The figure shows three views and two pictorial views of one solid part (mm, origin at its lowest corner). Answer the questions. A direction names the side the tool comes from. Round coordinates to 2 decimals unless told otherwise and drop trailing zeros. Order: outer loops, then holes, each group sorted by start corner. A loop starts at its lowest first (then second) coordinate and runs counter-clockwise, first axis right, second up. Notation, with made-up numbers: (28, 11) - (80, 11) arc R15 cw to (80, 39) - close; hole circle Ø6 at (-12, -26.75). An arc over 180 degrees is marked (long way). Answer in a Markdown table with one row per item.
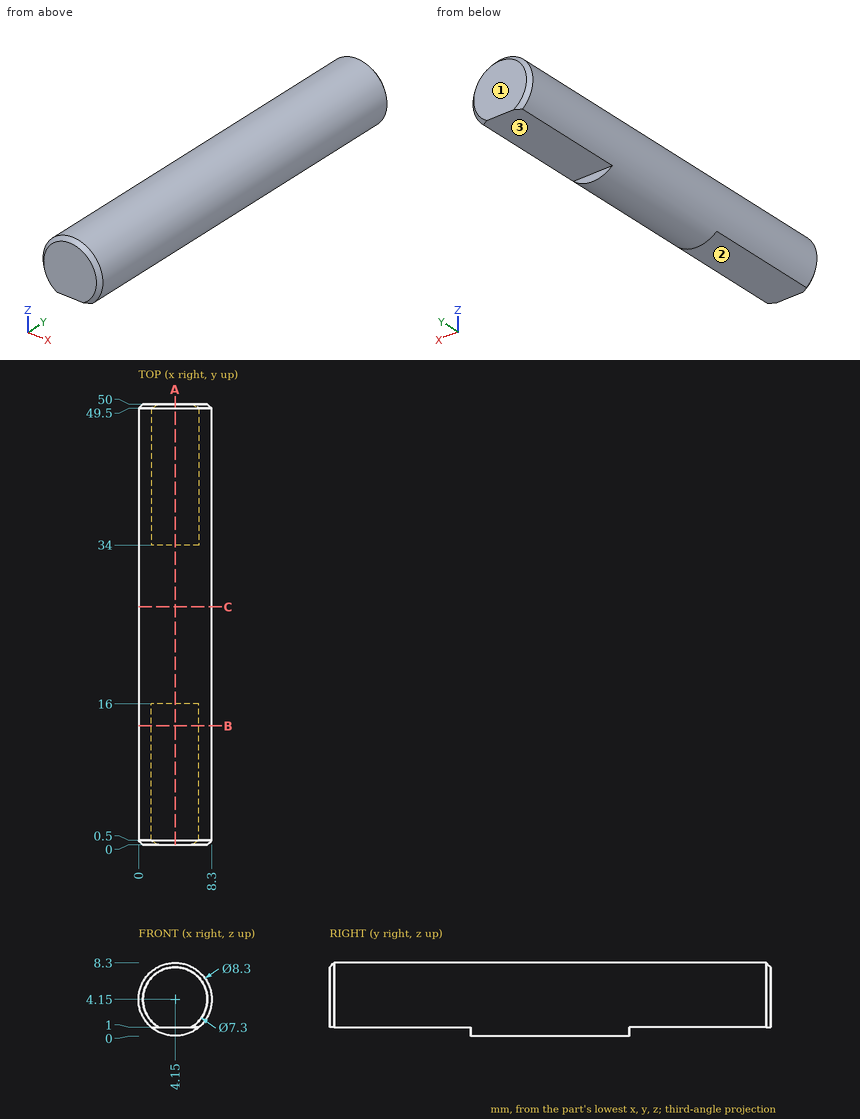
1) Which of the six approach directions +Z, -Z, +X, -X, +Y, -Y give full straight-line access (tool end or side, diameter ignored) to the marked faces 1, 2 and 3?
Filled in:
| item | result |
|---|---|
| face 1 | +Z, -Z, +X, -X, +Y |
| face 2 | -Z, +X, -X, -Y |
| face 3 | -Z, +X, -X, +Y |
2) Find section C-C, the plane y = 27. Give the vertices of the cut face in (x, z), then the cut area to 3 significant figures.
Filled in:
| item | result |
|---|---|
| outline | circle Ø8.3 at (4.15, 4.15) |
| area | 54.1 mm^2 |
3) Find section A-A, the plane x = 4.15. Give the vertices of the cut face in (y, z).
Filled in:
| item | result |
|---|---|
| outline | (0, 1) - (16, 1) - (16, 0) - (34, 0) - (34, 1) - (50, 1) - (50, 7.8) - (49.5, 8.3) - (0.5, 8.3) - (0, 7.8) - close |
4) Find section B-B, the plane y = 13.5. Give the vertices of the cut face in (x, z).
Filled in:
| item | result |
|---|---|
| outline | (1.45, 1) - (6.85, 1) arc R4.15 ccw (long way) to start |
5) Each of these flat-tipped pins is pushed along its axis until it touches: pin 1 (1 mm diameter, centred on y = 24.5, z = 1.5, fed in from -X); pin 2 (2 mm diameter, centred on y = 45, z = 4.5, fed in from +X); pin 3 (0.5 mm diameter, centred on x = 5, z = 0.5, fed in from +Y); pin 4 (4.5 mm diameter, centred on x = 4.5, y = 4, fed in from -Z). Where does it stop, or does it pass through?
Filled in:
| item | result |
|---|---|
| pin 1 | stops at x = 0.6 |
| pin 2 | stops at x = 8.3 |
| pin 3 | stops at y = 34 |
| pin 4 | stops at z = 1 |
6) Find the intervals of material crossed by probe 1 along X at (y, z) = (43, 4); probe 2 along X at (y, z) = (4, 5.5), in increasing order. Write a range as from..to.
Filled in:
| item | result |
|---|---|
| probe 1 | x = 0..8.3 |
| probe 2 | x = 0.23..8.07 |
